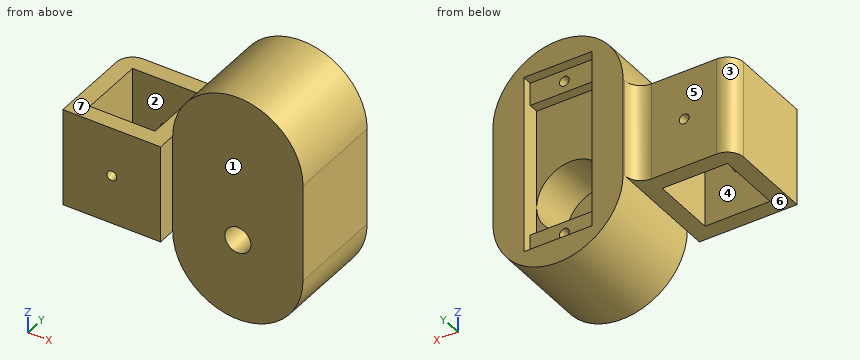
from build123d import *

# Parameters (mm, degrees)
SKETCH1_W           = 30
SKETCH1_H           = 30
SKETCH1_W_2         = 20
SKETCH1_H_2         = 20
BOSS_EXTRUDE2_DEPTH = 30
BOSS_EXTRUDE3_DEPTH = 30
SKETCH6_W           = 21
SKETCH6_H           = 55
CUT_EXTRUDE1_DEPTH  = 3
SKETCH7_R           = 1.5
CUT_EXTRUDE2_DEPTH  = 5
SKETCH8_W           = 21
SKETCH8_H           = 40.9
CUT_EXTRUDE3_DEPTH  = 3
SKETCH9_R           = 10.5
CUT_EXTRUDE4_DEPTH  = 81.056214629
BOSS_EXTRUDE4_START = -10
SKETCH10_R          = 10.5
SKETCH10_R_2        = 4
BOSS_EXTRUDE4_DEPTH = 10
FILLET1_DEPTH       = 30
FILLET1_2_DEPTH     = 30
SKETCH11_R          = 1.5
CUT_EXTRUDE6_DEPTH  = 81.175402093


with BuildPart() as part:
    # Sketch1 → Boss-Extrude2 (new body)
    with BuildSketch(Plane.XY):
        Rectangle(SKETCH1_W, SKETCH1_H)
        Rectangle(SKETCH1_W_2, SKETCH1_H_2, mode=Mode.SUBTRACT)
    extrude(amount=BOSS_EXTRUDE2_DEPTH)

    # Sketch5 → Boss-Extrude3 (add)
    with BuildSketch(Plane(origin=(0, 20.68, 0), x_dir=(1, 0, 0), z_dir=(0, 1, 0))):
        with BuildLine():
            Line((15, -30.030941434), (15, -0.030941434))
            ThreePointArc((15, -0.030941434), (35, 19.969058566), (55, -0.030941434))
            Line((55, -0.030941434), (55, -30.030941434))
            ThreePointArc((55, -30.030941434), (35, -50.030941434), (15, -30.030941434))
        make_face()
    extrude(amount=-BOSS_EXTRUDE3_DEPTH)

    # Sketch6 → Cut-Extrude1 (cut)
    with BuildSketch(Plane(origin=(0, 20.68, 0), x_dir=(1, 0, 0), z_dir=(0, 1, 0))):
        with Locations((35, -15.030941434)):
            Rectangle(SKETCH6_W, SKETCH6_H)
    extrude(amount=-CUT_EXTRUDE1_DEPTH, mode=Mode.SUBTRACT)

    # Sketch7 → Cut-Extrude2 (cut)
    with BuildSketch(Plane(origin=(0, 17.68, 0), x_dir=(1, 0, 0), z_dir=(0, 1, 0))):
        with Locations(Location((35, -39.030941434, 0), (0, 0, 270))):
            Circle(SKETCH7_R)
        with Locations(Location((35, 8.969058566, 0), (0, 0, 270))):
            Circle(SKETCH7_R)
    extrude(amount=-CUT_EXTRUDE2_DEPTH, mode=Mode.SUBTRACT)

    # Sketch8 → Cut-Extrude3 (cut)
    with BuildSketch(Plane(origin=(0, 17.68, 0), x_dir=(1, 0, 0), z_dir=(0, 1, 0))):
        with Locations((35, -15.030941434)):
            Rectangle(SKETCH8_W, SKETCH8_H)
    extrude(amount=-CUT_EXTRUDE3_DEPTH, mode=Mode.SUBTRACT)

    # Sketch9 → Cut-Extrude4 (cut, through all)
    with BuildSketch(Plane(origin=(0, 14.68, 0), x_dir=(1, 0, 0), z_dir=(0, 1, 0))):
        with Locations(Location((35, -5.030941434, 0), (0, 0, 270))):
            Circle(SKETCH9_R)
    extrude(amount=-CUT_EXTRUDE4_DEPTH, mode=Mode.SUBTRACT)

    # Sketch10 → Boss-Extrude4 (add)
    with BuildSketch(Plane.XZ.offset(9.32).offset(BOSS_EXTRUDE4_START)):
        with Locations(Location((35, 5.030941434, 0), (0, 0, 180))):
            Circle(SKETCH10_R)
        with Locations(Location((35, 5.030941434, 0), (0, 0, 270))):
            Circle(SKETCH10_R_2, mode=Mode.SUBTRACT)
    extrude(amount=BOSS_EXTRUDE4_DEPTH)

    # Fillet1: read off the stored shape, not the designer's step
    # Fillet1 outline → Fillet1 (cut)
    with BuildSketch(Plane.XY):
        with BuildLine():
            ThreePointArc((-15, 10), (-13.535533906, 13.535533906), (-10, 15))
            Line((-10, 15), (-15, 15))
            Line((-15, 15), (-15, 10))
        make_face()
    extrude(amount=FILLET1_DEPTH, mode=Mode.SUBTRACT)

    # Fillet1 2 outline → Fillet1 2 (add)
    with BuildSketch(Plane.XY):
        with BuildLine():
            ThreePointArc((15, 20), (13.535533906, 16.464466094), (10, 15))
            Line((10, 15), (15, 15))
            Line((15, 15), (15, 20))
        make_face()
    extrude(amount=FILLET1_2_DEPTH)

    # Sketch11 → Cut-Extrude6 (cut, through all)
    with BuildSketch(Plane(origin=(0, 15, 0), x_dir=(1, 0, 0), z_dir=(0, 1, 0))):
        with Locations(Location((0, -15, 0), (0, 0, 270))):
            Circle(SKETCH11_R)
    extrude(amount=-CUT_EXTRUDE6_DEPTH, mode=Mode.SUBTRACT)


solid = part.part
Here's how the part is built. I have some questions about the finished solid (model axes, mm). Face numbers are marked on the shaded views. A direction names the side the tool comes from. Round coordinates to 2 decimals unless told otherwise and drop trailing zeros. Order: outer loops, then holes, each group sorted by start corner. A loop starts at its lowest first (then second) coordinate and runs counter-clockwise, first axis right, second up. Notation, with made-up numbers: M 6,24.25 L 15,24.25 A21 cw 15,50.25 Z; hole C 56,5.25 d6. An arc over 180 degrees is marked long. One line per question, with ' | ' between items.
1) Imagine slicing it at B-B, the plane y = -0.5. Count the separate pieces of the cut face and the enclosed holes in it, plus the area to 3 significant figures.
Checked values:
separate pieces: 2 | enclosed holes: 1 | area: 2,710 mm²
2) On a 3-axis mill with a long thin cutter (end or side, diameter ignored), from which of +Z, -Z, +X, -X, +Y, -Y can I reach the whole of each face in a straight line? I mean the marked faces 4, 5, 6 and 7. Say none if no direction works.
Checked values:
face 4: +Z, -Z | face 5: +Z, -Z, -X, +Y | face 6: -Z, -X, +Y, -Y | face 7: +Z, -X, +Y, -Y
3) Imagine slicing it at C-C, the plane z = 19. Write out the boundary of the cut face in (x, y), plus the area to 3 significant figures.
Checked values:
outline: M -15,-15 L 15,-15 L 15,-9.32 L 55,-9.32 L 55,20.68 L 45.5,20.68 L 45.5,14.68 L 24.5,14.68 L 24.5,20.68 L 15,20.68 L 15,20 A5 cw 10,15 L -10,15 A5 ccw -15,10 Z; hole M -10,-10 L 10,-10 L 10,10 L -10,10 Z | area: 1,570 mm²
4) Imagine slicing it at A-A, the plane x = 35. Write out the boundary of the cut face in (y, z), plus the area to 3 significant figures.
Checked values:
outline: M -9.32,-19.97 L 20.68,-19.97 L 20.68,-12.47 L 17.68,-12.47 L 17.68,-10.47 L 12.68,-10.47 L 12.68,-7.47 L 17.68,-7.47 L 17.68,-5.42 L 14.68,-5.42 L 14.68,-5.47 L 0.68,-5.47 L 0.68,1.03 L -9.32,1.03 Z; M -9.32,9.03 L 0.68,9.03 L 0.68,15.53 L 14.68,15.53 L 14.68,35.48 L 17.68,35.48 L 17.68,37.53 L 12.68,37.53 L 12.68,40.53 L 17.68,40.53 L 17.68,42.53 L 20.68,42.53 L 20.68,50.03 L -9.32,50.03 Z | area: 1,410 mm²
5) We'd pull the mould along X, two halves only. Please class the marked faces 1, 2 and 3: released by +X, released by -X, zero draft, split by the parting line, or undercut.
Checked values:
face 1: zero draft | face 2: undercut | face 3: released by -X
6) Imagine slicing it at D-D, the plane x = 0. Write out the boundary of the cut face in (y, z).
Checked values:
outline: M -15,0 L -10,0 L -10,13.5 L -15,13.5 Z; M -15,16.5 L -10,16.5 L -10,30 L -15,30 Z; M 10,0 L 15,0 L 15,13.5 L 10,13.5 Z; M 10,16.5 L 15,16.5 L 15,30 L 10,30 Z
7) I need wall thicknesses on line 1 (X direction, y = -11.4, z = 15); line 2 (Y direction, x = -4, z = 12); line 3 (Z direction, x = 35, y = 4.75). Which ranges of each line are inside material? Lowest first, please.
Checked values:
line 1: x = -15 to -1.5, 1.5 to 15 | line 2: y = -15 to -10, 10 to 15 | line 3: z = -19.97 to -5.47, 15.53 to 50.03
8) I'm going to push flat-ended pins straight in: pin 1 Ø5 at (x, z) = (31, 18) entering from -Y; pin 2 Ø12 at (y, z) = (16, 20) entering from -X; pin 3 Ø2.5 at (x, y) = (30, 15.5) entering from -Z; pin 4 Ø16 at (x, z) = (-4, 20) entering from +Y. Where does each tip first touch, or does it pass through?
Checked values:
pin 1: stops at y = -9.32 | pin 2: stops at x = -15 | pin 3: stops at z = -19.61 | pin 4: stops at y = 15
